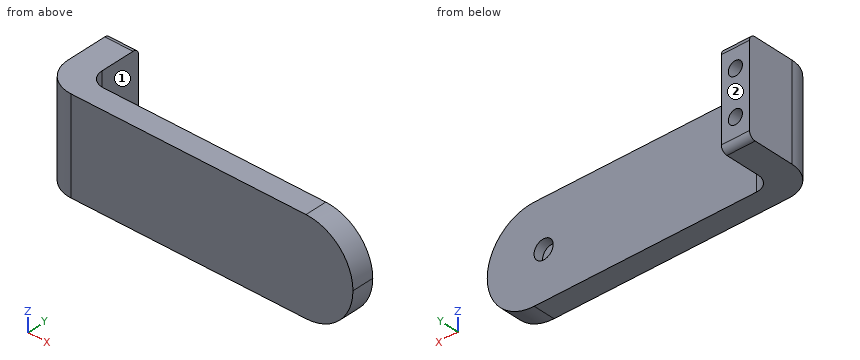
```python
from build123d import *

# Parameters (mm, degrees)
BOSS_EXTRUDE1_DEPTH = 30
SKETCH2_R           = 2.25
CUT_EXTRUDE1_DEPTH  = 6
FILLET1_R           = 5
FILLET2_R           = 10
SKETCH3_R           = 3.05
CUT_EXTRUDE3_DEPTH  = 3
FILLET3_R           = 15
FILLET4_R           = 2


with BuildPart() as part:
    # Sketch1 → Boss-Extrude1 (new body)
    with BuildSketch(Plane.XY):
        Polygon((-4.5, 21.5), (4.5, 21.5), (4.5, 3.5), (95.5, 3.5), (95.5, -3.5), (-4.5, -3.5), align=None)
    extrude(amount=BOSS_EXTRUDE1_DEPTH)

    # Sketch2 → Cut-Extrude1 (cut)
    with BuildSketch(Plane(origin=(0, 21.5, 0), x_dir=(1, 0, 0), z_dir=(0, 1, 0))):
        with Locations(Location((0, -22, 0), (0, 0, 270))):
            Circle(SKETCH2_R)
        with Locations(Location((0, -8, 0), (0, 0, 270))):
            Circle(SKETCH2_R)
    extrude(amount=-CUT_EXTRUDE1_DEPTH, mode=Mode.SUBTRACT)

    # Fillet1
    fillet1_edges = [part.edges().sort_by_distance(p)[0] for p in [
        (4.5, 3.5, 15),
    ]]
    fillet(fillet1_edges, radius=FILLET1_R)

    # Fillet2
    fillet2_edges = [part.edges().sort_by_distance(p)[0] for p in [
        (-4.5, -3.5, 15),
    ]]
    fillet(fillet2_edges, radius=FILLET2_R)

    # Sketch3 → Cut-Extrude3 (cut)
    with BuildSketch(Plane.XZ.offset(-3.5)):
        with Locations((77.5, 15)):
            Circle(SKETCH3_R)
    extrude(amount=CUT_EXTRUDE3_DEPTH, mode=Mode.SUBTRACT)

    # Fillet3
    fillet3_edges = [part.edges().sort_by_distance(p)[0] for p in [
        (95.5, 0, 30),
        (95.5, 0, 0),
    ]]
    fillet(fillet3_edges, radius=FILLET3_R - 0.0001)  # a hair under: the kernel refuses the full size

    # Fillet4
    fillet4_edges = [part.edges().sort_by_distance(p)[0] for p in [
        (0, 21.5, 30),
        (0, 21.5, 0),
    ]]
    fillet(fillet4_edges, radius=FILLET4_R)


solid = part.part
```
Build history of the part. All positions in model axes, mm. Face numbers are marked on the shaded views. A direction names the side the tool comes from. Coordinates: 2 decimals unless noted, no trailing zeros. Write each loop counter-clockwise with the first axis right and the second up, starting at its lowest first coordinate (ties: lowest second). Pieces come first, ordered by that corner, then holes.
1. Drop flat-ended pins along their axis: pin 1 (6.5 mm diameter, centred on y = 14, z = 18.5, fed in from +X); pin 2 (4 mm diameter, centred on x = 38, y = 6, fed in from -Z); pin 3 (8 mm diameter, centred on x = 77.5, z = 15, fed in from +Y); pin 4 (8 mm diameter, centred on x = 31.5, y = 5.5, fed in from +Z). Give the stop position or say it passes through.
Answer block:
pin 1: stops at x = 4.5
pin 2: passes through
pin 3: stops at y = 3.5
pin 4: stops at z = 30
2. Band-saw the part on A-A, the plane x = 77.5. Give the cut face in (y, z), and give its area (3 significant figures).
Answer block:
outline: (-3.5, 0) - (3.5, 0) - (3.5, 11.95) - (0.5, 11.95) - (0.5, 18.05) - (3.5, 18.05) - (3.5, 30) - (-3.5, 30) - close
area: 192 mm2
3. 3-axis set-ups, long thin cutter, end or side, ignore diameter. For the marked faces 1 and 2: which of +Z, -Z, +X, -X, +Y, -Y reach the whole face in a straight line?
Answer block:
face 1: +Z, -Z, +X, +Y
face 2: +Z, -Z, +X, -X, +Y
4. Band-saw the part on D-D, the plane x = 0. Give the cut face in (y, z).
Answer block:
outline: (-1.85, 0) - (19.5, 0) arc R2 ccw to (21.5, 2) - (21.5, 5.75) - (15.5, 5.75) - (15.5, 10.25) - (21.5, 10.25) - (21.5, 19.75) - (15.5, 19.75) - (15.5, 24.25) - (21.5, 24.25) - (21.5, 28) arc R2 ccw to (19.5, 30) - (-1.85, 30) - close
5. Drill centre lines: probe 1 along X at (y, z) = (17.85, 8); probe 2 along X at (y, z) = (15.5, 2.5); probe 3 along Y at (x, z) = (5.5, 26). Where is each one in solid material? Low to high.
Answer block:
probe 1: x = -4.5 to -2.25, 2.25 to 4.5
probe 2: x = -4.5 to 4.5
probe 3: y = -3.5 to 5.5
6. Band-saw the part on B-B, the plane z = 7. Give the cut face in (x, y), and give its area (3 significant figures).
Answer block:
outline: (-4.5, 6.5) arc R10 ccw to (5.5, -3.5) - (93.19, -3.5) - (93.19, 3.5) - (9.5, 3.5) arc R5 cw to (4.5, 8.5) - (4.5, 21.5) - (2.02, 21.5) - (2.02, 15.5) - (-2.02, 15.5) - (-2.02, 21.5) - (-4.5, 21.5) - close
area: 806 mm2
